from build123d import *

# Parameters (mm, degrees)
SKETCH1_W             = 30
SKETCH1_H             = 52
BASE_EXTRUDE_DEPTH    = 7
SKETCH2_W             = 30
SKETCH2_H             = 35
CUT_EXTRUDE1_DEPTH    = 15
SKETCH3_R             = 3.175
CUT_EXTRUDE2_DEPTH    = 15
F_8_CLEARANCE_HOLE1_D = 4.3053
SKETCH6_W             = 10
SKETCH6_H             = 14
CUT_EXTRUDE3_DEPTH    = 7
FILLET1_R             = 1


with BuildPart() as part:
    # Sketch1 → Base-Extrude (new body, symmetric)
    with BuildSketch(Plane.XY):
        Rectangle(SKETCH1_W, SKETCH1_H)
    extrude(amount=BASE_EXTRUDE_DEPTH, both=True)

    # Sketch2 → Cut-Extrude1 (cut, through all)
    with BuildSketch(Plane.XY.offset(7)):
        with Locations((0, 8.5)):
            Rectangle(SKETCH2_W, SKETCH2_H)
    extrude(amount=-CUT_EXTRUDE1_DEPTH, mode=Mode.SUBTRACT)

    # Sketch3 → Cut-Extrude2 (cut, through all)
    with BuildSketch(Plane.XY.offset(7)):
        with Locations((0, -15)):
            Circle(SKETCH3_R)
    extrude(amount=-CUT_EXTRUDE2_DEPTH, mode=Mode.SUBTRACT)

    # #8 Clearance Hole1 (through all)
    with Locations(Plane(origin=(-8.315488936, -9, -4.532476802), x_dir=(-1, 0, 0), z_dir=(0, 1, 0))):
        with Locations((-18.315488936, 4.532476802), (1.684511064, 4.532476802)):
            Hole(F_8_CLEARANCE_HOLE1_D / 2)

    # Sketch6 → Cut-Extrude3 (cut)
    with BuildSketch(Plane(origin=(0, -9, 0), x_dir=(-1, 0, 0), z_dir=(0, 1, 0))):
        with Locations((10, 0)):
            Rectangle(SKETCH6_W, SKETCH6_H)
        with Locations((-10, 0)):
            Rectangle(SKETCH6_W, SKETCH6_H)
    extrude(amount=-CUT_EXTRUDE3_DEPTH, mode=Mode.SUBTRACT)

    # Fillet1
    fillet1_edges = [part.edges().sort_by_distance(p)[0] for p in [
        (-5, -9, 0),
        (-5, -16, 0),
        (5, -9, 0),
        (5, -16, 0),
    ]]
    fillet(fillet1_edges, radius=FILLET1_R)


solid = part.part
Input: part model. Units: mm. Frame: model coordinates. A direction names the side the tool comes from. Coordinates: 2 decimals unless noted, no trailing zeros. Loops run counter-clockwise (first coordinate to the right, second up) from the corner with the lowest first, then second, coordinate; pieces in that order, holes last.
(1) Set-up query: faces 4 (the face through (0, -19, -7)), 5 (the face through (-12.4, -16, 0.1)), 6 (the face through (12, -16, 2)). Return all of +Z, -Z, +X, -X, +Y, -Y with unobstructed straight access to the full face (end or side cutting, diameter ignored); none if empty.
(2) Pull-direction query (X, two-part tool) for faces 1 (the face through (5, -12, 0)), 2 (the face through (12.053, -21.07, 0.647)), 3 (the face through (-5, -12, 0)); classes: released by +X, released by -X, zero draft, split by the parting line, or undercut.
(3) Material intervals for probe 1 along Z at (x, y) = (-10, -23); probe 2 along Y at (x, z) = (0, 3.5) (3 decimals); probe 3 along Y at (x, z) = (13.5, 3.5), sorted ascending.
(4) Section D-D on y = -12.25. Return the cut outline in (x, z), then the cut area to 3 significant figures.
(5) Section B-B on x = 10. Return the cut outline in (y, z), then the cut area to 3 significant figures.
(6) Section C-C on z = -2.5. Return the cut outline in (x, y) (3 decimals), then the cut area to 3 significant figures.
(7) Section A-A on z = 0. Return the cut outline in (x, y) (3 decimals).
(8) First-contact query: pin 1 Ø2.5 at (x, z) = (12.5, -3) entering from +Y; pin 2 Ø2.5 at (x, z) = (-10, 0) entering from -Y; pin 3 Ø1.5 at (y, z) = (-11.5, 0) entering from -X; pin 4 Ø2 at (y, z) = (-14.5, 1.5) entering from -X. Flat tips, straight axial feed; report the tip coordinate or a pass-through.
Data:
1. face 4: -Z, +X, -X, +Y, -Y
1. face 5: +Z, -Z, -X, +Y
1. face 6: +Z, -Z, +X, +Y
2. face 1: released by +X
2. face 2: undercut
2. face 3: released by -X
3. probe 1: z = -7 to -2.15, 2.15 to 7
3. probe 2: y = -26 to -18.175, -11.825 to -9
3. probe 3: y = -26 to -16
4. outline: (-5, -7) - (-1.59, -7) - (-1.59, 7) - (-5, 7) - close; (1.59, -7) - (5, -7) - (5, 7) - (1.59, 7) - close
4. area: 95.6 mm2
5. outline: (-26, -7) - (-16, -7) - (-16, -2.15) - (-26, -2.15) - close; (-26, 2.15) - (-16, 2.15) - (-16, 7) - (-26, 7) - close
5. area: 96.9 mm2
6. outline: (-15, -26) - (15, -26) - (15, -16) - (6, -16) arc R1 cw to (5, -15) - (5, -10) arc R1 ccw to (4, -9) - (-4, -9) arc R1 ccw to (-5, -10) - (-5, -15) arc R1 cw to (-6, -16) - (-15, -16) - close; hole circle Ø6.35 at (0, -15)
6. area: 338 mm2
7. outline: (-15, -26) - (-12.153, -26) - (-12.153, -16) - (-15, -16) - close; (-7.847, -26) - (7.847, -26) - (7.847, -16) - (6, -16) arc R1 cw to (5, -15) - (5, -10) arc R1 ccw to (4, -9) - (-4, -9) arc R1 ccw to (-5, -10) - (-5, -15) arc R1 cw to (-6, -16) - (-7.847, -16) - close; (12.153, -26) - (15, -26) - (15, -16) - (12.153, -16) - close; hole circle Ø6.35 at (0, -15)
8. pin 1: stops at y = -16
8. pin 2: passes through
8. pin 3: stops at x = -5
8. pin 4: stops at x = -5.13
